Can you work these out from the model? Positions are in its coordinate system, mm. A direction names the side the tool comes from. Give positions to 0.01 mm unless a question says otherwise; leave off trailing zeros. Write each loop counter-clockwise with the first axis right and the second up, starting at its lowest first coordinate (ties: lowest second). Pieces come first, ordered by that corner, then holes. Notation, with made-up numbers: (53.5, 24) -> (111.5, 24) arc R19 cw to (111.5, 42) -> close; hole circle Ø5 at (20, 75.25). An arc over 180 degrees is marked (long way). One line per item, written item: value.
Autodesk Inventor part; units mm, degrees
ref_plane "YZ Plane" through (0, 0, 0) normal (1, 0, 0) x (0, 1, 0)
ref_plane "XZ Plane" through (0, 0, 0) normal (0, 1, 0) x (-1, 0, 0)
ref_plane "XY Plane" through (0, 0, 0) normal (0, 0, 1) x (1, 0, 0)
sketch "Sketch1" plane through (0, 0, 0) normal (0, 0, 1) x (1, 0, 0)
  line L0 (-20, -5) -> (20, -5)
  line L1 (20, -5) -> (20, 5)
  line L2 (20, 5) -> (-20, 5)
  line L3 (-20, 5) -> (-20, -5)
  line L4 (-20, -5) -> (20, 5) construction
  line L5 (20, -5) -> (-20, 5) construction
  circle A0 centre (0, -18) radius 11.15
  circle A1 centre (0, -18) radius 5.25
  circle A2 centre (0, -18) radius 17.5
  line L6 (-20, -5) -> (-17.2455, -20.9738)
  line L7 (20, -5) -> (17.2455, -20.9738)
  circle A3 centre (0, -10) radius 1.65
  circle A4 centre (-8, -18) radius 1.65
  circle A5 centre (0, -26) radius 1.65
  circle A6 centre (8, -18) radius 1.65
  circle A7 centre (34, -18) radius 7.65
  line L8 (21.5, -30.5) -> (46.5, -30.5)
  line L9 (46.5, -30.5) -> (46.5, -5.5)
  line L10 (46.5, -5.5) -> (21.5, -5.5)
  line L11 (21.5, -5.5) -> (21.5, -30.5)
  line L12 (21.5, -30.5) -> (46.5, -5.5) construction
  line L13 (46.5, -30.5) -> (21.5, -5.5) construction
  circle A8 centre (25.5, -9.5) radius 1.65
  circle A9 centre (42.5, -9.5) radius 1.65
  circle A10 centre (42.5, -26.5) radius 1.65
  circle A11 centre (25.5, -26.5) radius 1.65
  line L14 (46.5, -5.5) -> (20, 0)
  line L15 (21.5, -30.5) -> (4.396, -34.9389)
  line L16 (0, 5) -> (0, 15.3431)
  circle A12 centre (-34, -18) radius 7.65
  line L17 (-21.5, -30.5) -> (-46.5, -30.5)
  line L18 (-46.5, -30.5) -> (-46.5, -5.5)
  line L19 (-46.5, -5.5) -> (-21.5, -5.5)
  line L20 (-21.5, -5.5) -> (-21.5, -30.5)
  line L21 (-21.5, -30.5) -> (-46.5, -5.5) construction
  line L22 (-46.5, -30.5) -> (-21.5, -5.5) construction
  circle A13 centre (-25.5, -9.5) radius 1.65
  circle A14 centre (-42.5, -9.5) radius 1.65
  circle A15 centre (-42.5, -26.5) radius 1.65
  circle A16 centre (-25.5, -26.5) radius 1.65
  line L23 (-46.5, -5.5) -> (-20, 0)
  line L24 (-21.5, -30.5) -> (-4.396, -34.9389)
  point P0 (0, 0)
  point P1 (-4.396, -34.9389)
  dimension "d0" = 22.3
  dimension "d1" = 10.5
  dimension "d2" = 35
  dimension "d3" = 3.3
  dimension "d4" = 8
  dimension "d7" = 360
  dimension "d14" = 40
  dimension "d16" = 23
  dimension "d17" = 10
  dimension "d24" = 15.3
  dimension "d25" = 34
  dimension "d27" = 25
  dimension "d28" = 25
  dimension "d29" = 3.3
  dimension "d30" = 17
extrude "Extrusion1" add sketch "Sketch1" along normal blind 10 contours L3 L2 L1 L0 A2 | L0 A2 L6 | A2 L0 | L0 A2 | L0 L7 A2 | A0
extrude "Extrusion2" cut sketch "Sketch1" along normal blind 3 contours A0
extrude "Extrusion4" add sketch "Sketch1" along normal blind 10 contours L6 A2 L24 L20 L19 L23 L3 | L19 L20 L17 L18 | L1 L14 L10 L11 L15 A2 L7 | L11 L10 L9 L8
fillet "Fillet1" radius 5 4 edges at (-46.5, -5.5, 5) (-46.5, -30.5, 5) (46.5, -30.5, 5) (46.5, -5.5, 5)
sketch "Sketch4" plane through (-20, 5, 0) normal (0, 1, 0) x (1, 0, 0)
  line L0 (40, 0) -> (0, 0)
  line L1 (0, 0) -> (0, -10)
  line L2 (40, -10) -> (0, -10)
  line L3 (40, 0) -> (40, -10)
  point P0 (20, 0)
extrude "Extrusion5" add sketch "Sketch4" along normal blind 5.5
sketch "Sketch5" plane through (-20, 10.5, 0) normal (0, 1, 0) x (1, 0, 0)
  line L0 (40, 0) -> (0, 0)
  line L1 (0, 0) -> (0, -10)
  line L2 (0, -10) -> (40, -10)
  line L3 (40, -10) -> (40, 0)
  line L4 (40, 0) -> (0, -10)
  line L5 (0, 5) -> (40, 5)
  line L6 (40, 5) -> (40, -15)
  line L7 (40, -15) -> (0, -15)
  line L8 (0, -15) -> (0, 5)
  line L9 (0, 5) -> (40, -15) construction
  line L10 (40, 5) -> (0, -15) construction
  point P0 (20, 0)
  point P1 (20, -5)
extrude "Extrusion6" add sketch "Sketch5" against normal blind 10.5
chamfer "Chamfer1" distance 5 angle 45 2 edges at (0, 0, 10) (0, 0, 0)
sketch "Sketch7" plane through (-20, 10.5, 0) normal (0, 1, 0) x (1, 0, 0)
  line L0 (0, 5) -> (0, -15)
  line L1 (0, -15) -> (40, -15)
  line L2 (40, -15) -> (40, 5)
  line L3 (40, 5) -> (0, 5)
  line L4 (0, -5) -> (40, -5)
  line L5 (20, -5) -> (34, -5)
  line L6 (34, -5) -> (25, -5)
  circle A0 centre (34, -5) radius 2
  line L7 (34, -5) -> (25, -5)
  circle A1 centre (25, -5) radius 2
  line L8 (20, -5) -> (20, -8)
  circle A2 centre (6, -5) radius 2
  circle A3 centre (15, -5) radius 2
  point P0 (20, 0)
  dimension "d45" = 14
  dimension "d47" = 4
  dimension "d48" = 9
  dimension "d49" = 4
fillet "Fillet2" radius 15 2 edges at (-20, 0, 5) (20, 0, 5)
fillet "Fillet3" radius 5 2 edges at (0, 0, -5) (0, 0, 15)
extrude "Extrusion7" cut sketch "Sketch7" against normal blind 18 contours A2 L4 | L4 A2 | A0 L4 | L4 A0 | A3 L4 | L4 A3 | A1 L4 | L4 A1
properties part number "PARA_TUERCA" material "Steel, Mild, Welded"
1) If we section it at D-D (y = 0.5): Write out the boundary of the cut face in (x, z).
Answer list:
outline: (-25.55, -4.75) -> (25.55, -4.75) -> (25.55, 14.75) -> (-25.55, 14.75) -> close; hole circle Ø4 at (-14, 5); hole circle Ø4 at (-5, 5); hole circle Ø4 at (5, 5); hole circle Ø4 at (14, 5)
2) If we section it at C-C (z = 8.5): State how many separate pieces and enclosed holes the cut face has, and give its area (3 significant figures).
Answer list:
separate pieces: 1
enclosed holes: 15
area: 2,710 mm^2
3) If we section it at A-A (x = 0): Write out the boundary of the cut face in (y, z), and give its area (3 significant figures).
Answer list:
outline: (-35.5, 0) -> (-29.15, 0) -> (-29.15, 3) -> (-27.65, 3) -> (-27.65, 10) -> (-35.5, 10) -> close; (-24.35, 3) -> (-23.25, 3) -> (-23.25, 10) -> (-24.35, 10) -> close; (-12.75, 3) -> (-11.65, 3) -> (-11.65, 10) -> (-12.75, 10) -> close; (-8.35, 3) -> (-6.85, 3) -> (-6.85, 0) -> (-5, 0) -> (-1.46, -3.54) arc R5 ccw to (2.07, -5) -> (10.5, -5) -> (10.5, 15) -> (2.07, 15) arc R5 ccw to (-1.46, 13.54) -> (-5, 10) -> (-8.35, 10) -> close
area: 402 mm^2
4) We'd pull the mould along X, two halves only. Please class faces 1 (the face through (23.85, -9.57, 4.93)), 2 (the face through (-1, -3, -2)), 3 (the face through (46.5, -18, 5)), 4 (the face through (-37.259, -3.582, 4.894)): released by +X, released by -X, zero draft, split by the parting line, or undercut.
Answer list:
face 1: undercut
face 2: zero draft
face 3: released by +X
face 4: released by -X
5) I need wall thicknesses on L1, parallel to Y at x = 0, z = 6.5; L2, parallel to Z at x = -14, y = 2; L3, parallel to X at y = -24, z = 5. Which ranges of each line are inside material? Lowest first, please.
Answer list:
L1: y = -35.5 to -27.65, -24.35 to -23.25, -12.75 to -11.65, -8.35 to 10.5
L2: z = -5 to 3, 7 to 15
L3: x = -46.5 to -38.75, -29.25 to 29.25, 38.75 to 46.5
6) If we section it at B-B (y = -14): Write out the boundary of the cut face in (x, z).
Answer list:
outline: (-46.5, 0) -> (-40.52, 0) -> (-40.52, 10) -> (-46.5, 10) -> close; (-27.48, 0) -> (-10.41, 0) -> (-10.41, 3) -> (-3.4, 3) -> (-3.4, 10) -> (-27.48, 10) -> close; (3.4, 3) -> (10.41, 3) -> (10.41, 0) -> (27.48, 0) -> (27.48, 10) -> (3.4, 10) -> close; (40.52, 0) -> (46.5, 0) -> (46.5, 10) -> (40.52, 10) -> close
7) Will these pins go through, and if not, where does the flat tip stop? pin 1 (6.5 mm diameter, centred on x = -14, z = 5, fed in from +Y); pin 2 (8 mm diameter, centred on x = 2, y = -5.5, fed in from +Z); pin 3 (1.5 mm diameter, centred on x = -33, z = 2.5, fed in from -Y); pin 4 (3 mm diameter, centred on y = -5, z = 5.5, fed in from -X).
Answer list:
pin 1: stops at y = 10.5
pin 2: stops at z = 13.5
pin 3: stops at y = -30.5
pin 4: stops at x = -45.45
8) For faces 5 (the face through (-6.6, 1.6, 6.2)), 6 (the face through (31, -30.5, 5)), 7 (the face through (45, -6, 5)), 8 (the face through (6, -27.4, 1.5)), 9 (the face through (-23.743, 2.202, 4.86)), which set-ups out of +Z, -Z, +X, -X, +Y, -Y let a thin tool reach every point of the face, with its end or its side?
Answer list:
face 5: +Y
face 6: +Z, -Z, +X, -Y
face 7: +Z, -Z, +X, +Y
face 8: -Z
face 9: +Z, -Z, -X, +Y
